from build123d import *

# Parameters (mm, degrees)
BOSS_EXTRU_1_DEPTH      = 9
ESQUISSE2_W             = 19.623971562
ESQUISSE2_H             = 15.534154535
ESQUISSE2_R             = 3
ENL_V_MAT_EXTRU_1_DEPTH = 3
ENL_V_START             = -4
ESQUISSE3_W             = 11.267201257
ESQUISSE3_H             = 13.961169169
ESQUISSE3_R             = 3
ENL_V_MAT_EXTRU_2_DEPTH = 4
CHANFREIN1_SIZE         = 4
CHANFREIN1_SIZE_2       = 2.499477408


with BuildPart() as part:
    # Esquisse1 → Boss.-Extru.1 (new body)
    with BuildSketch(Plane.XY):
        Polygon((4.041451884, 0), (2.020725942, 3.5), (-2.020725942, 3.5), (-4.041451884, 0), (-2.020725942, -3.5), (2.020725942, -3.5), align=None)
    extrude(amount=BOSS_EXTRU_1_DEPTH)

    # Esquisse2 → Enlèv. mat.-Extru.1 (cut)
    with BuildSketch(Plane.XY.offset(9)):
        with Locations((0.327116653, -1.544441398)):
            Rectangle(ESQUISSE2_W, ESQUISSE2_H)
        Circle(ESQUISSE2_R, mode=Mode.SUBTRACT)
    extrude(amount=-ENL_V_MAT_EXTRU_1_DEPTH, mode=Mode.SUBTRACT)

    # Esquisse3 → Enlèv. mat.-Extru.2 (cut)
    with BuildSketch(Plane(origin=(0, 0, 0), x_dir=(-1, 0, 0), z_dir=(0, 0, -1)).offset(ENL_V_START)):
        with Locations((0.009770186, 0.039262349)):
            Rectangle(ESQUISSE3_W, ESQUISSE3_H)
        with Locations(Location((0, 0, 0), (0, 0, 180))):
            Circle(ESQUISSE3_R, mode=Mode.SUBTRACT)
    extrude(amount=ENL_V_MAT_EXTRU_2_DEPTH, mode=Mode.SUBTRACT)

    # Chanfrein1
    # the kernel refuses this chamfer: 4, 2.499477408 mm, written as the material it takes off along each edge
    with BuildSketch(Plane(origin=(0, 0, 0), x_dir=(1, 0, 0), z_dir=(0, 1, 0))) as chanfrein1_piece_1_section:
        Polygon((3, -CHANFREIN1_SIZE), (3 - CHANFREIN1_SIZE_2, 0), (3, 0), align=None)
    chanfrein1_piece_1 = revolve(axis=Axis((0, 0, 0), (0, 0, -1)), mode=Mode.PRIVATE)
    chanfrein1_piece_1 = split(chanfrein1_piece_1, bisect_by=Plane(origin=(-1.744026904, 0, 4), z_dir=(0, 0, -1)), keep=Keep.TOP, mode=Mode.PRIVATE)
    add(chanfrein1_piece_1, mode=Mode.SUBTRACT)

    # Esquisse4 → Enlèvement de matière-Révolution1 (revolve, cut)
    with BuildSketch(Plane(origin=(0, 0, 0), x_dir=(1, 0, 0), z_dir=(0, 1, 0))):
        Polygon((0, -9), (1, -9), (1, -1.642518405), (0.2, -0.5), (0.2, 0), (0, 0), align=None)
    revolve(axis=Axis((0, 0, 9.404603351), (0, 0, -1)), mode=Mode.SUBTRACT)


solid = part.part
Design review of the part built by this model. Coordinates are the model's own, in mm. A direction names the side the tool comes from. Round coordinates to 2 decimals unless told otherwise and drop trailing zeros. Loops run counter-clockwise (first coordinate to the right, second up) from the corner with the lowest first, then second, coordinate; pieces in that order, holes last. Notation, with made-up numbers: (78.5, 45.5) - (101.5, 45.5) arc R31 ccw to (101.5, 83.5) - close; hole circle Ø2 at (-8, -21). An arc over 180 degrees is marked (long way). One line per item, written item: value. Start each with the question number.
1) Consider section A-A on x = 0. Give the boundary of the cut face in (y, z).
2) To check wall thickness, follow L1, parallel to Y at x = 0, z = 5.75; L2, parallel to Y at x = 0, z = 7.75; L3, parallel to X at y = 0, z = 3.75. State the ranges of each line that lie inside material, in increasing order. Write a range as from..to.
3) Consider section C-C on z = 8. Give the boundary of the cut face in (x, y), then the cut area to 3 significant figures.
4) Consider section B-B on z = 5.5. Give the boundary of the cut face in (x, y), then the cut area to 3 significant figures.
5) Draft analysis for pull direction X (two halves, no side actions). For faces 4 (the conical face through (-0.1, 0.4, 0.8)), 5 (the cylindrical face through (0, 1, 5)), 6 (the flat face through (-1, 3, 6)), 7 (the flat face through (3.045, 1.726, 4.986)), state which applies: +X half, -X half, draft (parallel to the pull), parting line (faces both ways), or undercut.
6) For faces 1 (the cylindrical face through (-3, 0, 8)), 2 (the flat face through (0, 3.5, 5)), 3 (the flat face through (1, 3, 4)), list the 3-axis set-ups (+Z, -Z, +X, -X, +Y, -Y) from which the entire face can be reached by the end or side of a thin tool; tool diameter is ignored.
7) Insertion check: pin 1 Ø2 at (y, z) = (-0.5, 7.5) entering from +X; pin 2 Ø1.5 at (x, y) = (-3, -0.5) entering from -Z; pin 3 Ø2 at (y, z) = (1.5, 4) entering from -X. Each pin has a flat end and moves straight along its axis. Give the tip position at first contact, or say it passes through.
8) Consider section D-D on x = 3.75. Give the boundary of the cut face in (y, z), then the cut area to 3 significant figures.
Reported:
1. outline: (-3.5, 4) - (-3, 4) - (-0.5, 0) - (-0.2, 0) - (-0.2, 0.5) - (-1, 1.64) - (-1, 9) - (-3, 9) - (-3, 6) - (-3.5, 6) - close; (0.2, 0) - (0.5, 0) - (3, 4) - (3.5, 4) - (3.5, 6) - (3, 6) - (3, 9) - (1, 9) - (1, 1.64) - (0.2, 0.5) - close
2. L1: y = -3.5..-1, 1..3.5
2. L2: y = -3..-1, 1..3
2. L3: x = -2.84..-1, 1..2.84
3. outline: circle Ø6 at (0, 0); hole circle Ø2 at (0, 0)
3. area: 25.1 mm^2
4. outline: (-4.04, 0) - (-2.02, -3.5) - (2.02, -3.5) - (4.04, 0) - (2.02, 3.5) - (-2.02, 3.5) - close; hole circle Ø2 at (0, 0)
4. area: 39.3 mm^2
5. face 4: undercut
5. face 5: undercut
5. face 6: draft
5. face 7: +X half
6. face 1: +Z
6. face 2: +Z, -Z, +X, -X, +Y
6. face 3: -Z
7. pin 1: stops at x = 3
7. pin 2: stops at z = 2.87
7. pin 3: stops at x = -3.75
8. outline: (-0.5, 4) - (0.5, 4) - (0.5, 6) - (-0.5, 6) - close
8. area: 2.02 mm^2
